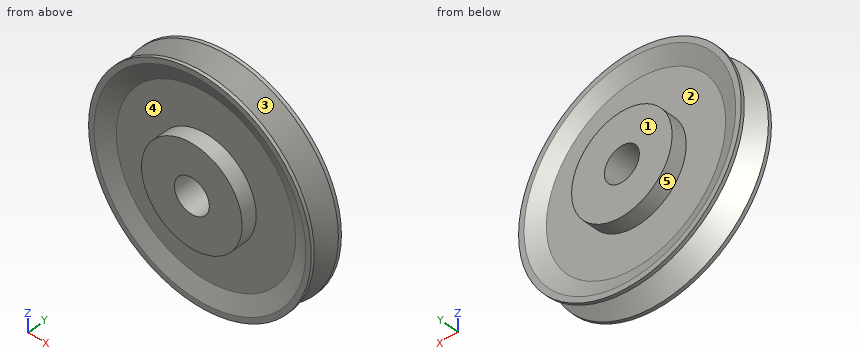
from build123d import *


with BuildPart() as part:
    # Sketch1 → Revolution1 (revolve)
    with BuildSketch(Plane.XY):
        Polygon((3.81, -1.828307296), (3.81, 0.457692704), (3.81, 2.235692704), (0, 2.235692704), (0, -3.606307296), (3.81, -3.606307296), align=None)
        Polygon((8.382, 0.457692704), (3.81, 0.457692704), (3.81, -1.828307296), (8.382, -1.828307296), (10.265714416, -2.590307296), (10.900714416, -2.590307296), (10.900714416, -2.209307296), (8.520461423, -0.685307296), (10.900714416, 0.838692704), (10.900714416, 1.219692704), (10.265714416, 1.219692704), align=None)
    revolve(axis=Axis((-2.032, -2.54, 0), (0, 1, 0)))


solid = part.part
Can you work these out from the model? Positions are in its coordinate system, mm. Face numbers are marked on the shaded views. A direction names the side the tool comes from. Round coordinates to 2 decimals unless told otherwise and drop trailing zeros. Loops run counter-clockwise (first coordinate to the right, second up) from the corner with the lowest first, then second, coordinate; pieces in that order, holes last. Notation, with made-up numbers: (-32.5, -0.75) - (20.5, -0.75) arc R32 ccw to (20.5, 29.25) - close; hole circle Ø11 at (-28, -34). An arc over 180 degrees is marked (long way). Answer in a Markdown table with one row per item. Add a question column.
Q1. For pin 1 Ø2 at (x, z) = (-11, -3) entering from -Y; pin 2 Ø3 at (y, z) = (1, -10) entering from -X; pin 3 Ø1 at (y, z) = (-2, 5.5) entering from +X, each with a flat end and sliding along its axis, tell me the tip position at first contact or that it passes through.
Q2. Which directions (+Z, -Z, +X, -X, +Y, -Y) give clear straight access to the entire face, cutting with the end or side of a thin tool? Please do the marked faces 3, 4 and 5.
Q3. I need wall thicknesses on L1, parallel to X at y = 0.85, z = 0; L2, parallel to Y at x = 3.5, z = 3; L3, parallel to X at y = 0.75, z = 0. Which ranges of each line are inside material? Lowest first, please.
Q4. I want a section at B-B on y = -1. List the corners of the cut face in (x, z) for me.
Q5. We'd pull the mould along Z, two halves only. Please class the marked faces 1 and 2: pulls with the +Z half, pulls with the -Z half, needs draft (parallel to the pull), parting line crosses it, or undercut.
A:
| question | item | result |
|---|---|---|
| 1 | pin 1 | y = -1.85 |
| 1 | pin 2 | x = -11.78 |
| 1 | pin 3 | x = 9.88 |
| 2 | face 3 | none |
| 2 | face 4 | -Y |
| 2 | face 5 | +Y |
| 3 | L1 | -14.96 to -13.42, -7.87 to -4.06, 0 to 3.81, 9.35 to 10.9 |
| 3 | L2 | -1.83 to 0.46 |
| 3 | L3 | -14.83 to -13.17, -7.87 to -4.06, 0 to 3.81, 9.1 to 10.76 |
| 4 | outline | circle Ø22.09 at (-2.03, 0); hole circle Ø4.06 at (-2.03, 0) |
| 5 | face 1 | needs draft |
| 5 | face 2 | undercut |
